from build123d import *

# Parameters (mm, degrees)
BOSS_EXTRUDE1_DEPTH = 25
SKETCH2_R           = 5
SKETCH2_W           = 17.097123546
SKETCH2_H           = 4.020670456
CUT_EXTRUDE1_DEPTH  = 100
BOSS_EXTRUDE2_DEPTH = 50


with BuildPart() as part:
    # Sketch1 → Boss-Extrude1 (new body)
    with BuildSketch(Plane.XY):
        Polygon((-120, 0), (-87.572195572, 56.166604847), (87.572195572, 56.166604847), (120, 0), (126.793465802, 0), (141.793465802, 0), (141.793465802, 5), (122.886751346, 5), (92.427804428, 57.756443607), (90.458946918, 61.166604847), (-90.458946918, 61.166604847), (-122.886751346, 5), (-141.793465802, 5), (-141.793465802, 0), (-126.793465802, 0), align=None)
    extrude(amount=BOSS_EXTRUDE1_DEPTH)

    # Sketch2 → Cut-Extrude1 (cut, symmetric)
    with BuildSketch(Plane(origin=(0, 5, 0), x_dir=(1, 0, 0), z_dir=(0, 1, 0))):
        with Locations((132.340108574, -12.5)):
            Circle(SKETCH2_R)
        with Locations((-132.340108574, -12.5)):
            Circle(SKETCH2_R)
        with Locations((0, -7.118249896)):
            Rectangle(SKETCH2_W, SKETCH2_H)
    extrude(amount=CUT_EXTRUDE1_DEPTH, both=True, mode=Mode.SUBTRACT)

    # Sketch3 → Boss-Extrude2 (add, symmetric)
    with BuildSketch(Plane(origin=(0, 0, 0), x_dir=(0, 0, -1), z_dir=(1, 0, 0))):
        Polygon((-30.808478502, 77.125268372), (-20.547874202, 48.934489749), (-25.246337306, 47.224389032), (-27.125722548, 46.540348745), (-28.493803121, 50.299119228), (-27.5541105, 50.641139372), (-26.52805007, 47.822061509), (-25.588357449, 48.164081653), (-35.164921463, 74.475475035), (-36.104614083, 74.133454891), (-35.078553653, 71.314377029), (-36.018246274, 70.972356886), (-37.386326847, 74.731127369), (-35.506941606, 75.415167656), align=None)
    extrude(amount=BOSS_EXTRUDE2_DEPTH, both=True)


solid = part.part
Verification items for the finished model (mm, model axes). A direction names the side the tool comes from. Coordinates: 2 decimals unless noted, no trailing zeros. Order: outer loops, then holes, each group sorted by start corner. A loop starts at its lowest first (then second) coordinate and runs counter-clockwise, first axis right, second up. Notation, with made-up numbers: M 30.25,-38 L 54.25,-38 A28 ccw 54.25,-8 Z; hole C 46.5,50 d9. An arc over 180 degrees is marked long. One line per item, written item: value. Start each with the question number.
Item 1: Sectioned sample at C-C (y = 22). Enter the section's corners in (x, z), then the cut area to 3 significant figures.
Item 2: Mould release check, pull along X, two halves, no side actions. Record for faces 1 (the flat face through (-104.013, 27.69, 12.325)), 2 (the flat face through (126, 0, 12)), 3 (the flat face through (-141.793, 3, 12)): released by +X, released by -X, zero draft, split by the parting line, or undercut.
Item 3: Sectioned sample at B-B (x = -30). Enter the section's corners in (y, z), then the cut area to 3 significant figures.
Item 4: Scan lines: probe 1 along Y at (x, z) = (52, 14); probe 2 along X at (y, z) = (4, 14.5); probe 3 along Y at (x, z) = (-16, 23.5). Record each from-to range of solid material in increasing order.
Item 5: Gauge pin test, flat ends, axial feed: pin 1 (5 mm diameter, centred on y = 64, z = 33, fed in from -X); pin 2 (2 mm diameter, centred on y = 59, z = 6.5, fed in from +X); pin 3 (5.5 mm diameter, centred on x = -129.5, z = 11.5, fed in from +Y); pin 4 (6 mm diameter, centred on x = -132.34, z = 12.5, fed in from -Y). Record the tip position at first contact, or that the pin passes through.
Item 6: Sectioned sample at D-D (y = 67). Enter the section's corners in (x, z).
Item 7: Access from +Z, -Z, +X, -X, +Y, -Y to the whole of each face (thin tool, end or side, straight path). Record for faces 4 (the flat face through (1, 61.167, 12)), 5 (the flat face through (137, 5, 10)), 6 (the flat face through (0.7, 52.6, 21.88)).
Item 8: Sectioned sample at A-A (z = 12.5). Enter the section's corners in (x, y).
Conclusion:
1. outline: M -113.07,0 L -107.3,0 L -107.3,25 L -113.07,25 Z; M 107.3,0 L 113.07,0 L 113.07,25 L 107.3,25 Z
1. area: 289 mm^2
2. face 1: undercut
2. face 2: zero draft
2. face 3: released by -X
3. outline: M 46.54,27.13 L 48.93,20.55 L 56.17,23.18 L 56.17,0 L 61.17,0 L 61.17,25 L 77.13,30.81 L 74.73,37.39 L 70.97,36.02 L 71.31,35.08 L 74.13,36.1 L 74.48,35.16 L 48.16,25.59 L 47.82,26.53 L 50.64,27.55 L 50.3,28.49 Z
3. area: 280 mm^2
4. probe 1: y = 56.17 to 61.17
4. probe 2: x = -141.79 to -136.92, -127.76 to -117.69, 117.69 to 127.76, 136.92 to 141.79
4. probe 3: y = 47.86 to 61.17
5. pin 1: stops at x = -50
5. pin 2: stops at x = 92.29
5. pin 3: stops at y = 5
5. pin 4: passes through
6. outline: M -50,27.12 L 50,27.12 L 50,32.44 L -50,32.44 Z
7. face 4: -Z, +X, -X, +Y
7. face 5: +Z, -Z, +X, +Y
7. face 6: -Z
8. outline: M -141.79,0 L -137.34,0 L -137.34,5 L -141.79,5 Z; M -127.34,0 L -120,0 L -87.57,56.17 L 87.57,56.17 L 120,0 L 127.34,0 L 127.34,5 L 122.89,5 L 90.46,61.17 L -90.46,61.17 L -122.89,5 L -127.34,5 Z; M 137.34,0 L 141.79,0 L 141.79,5 L 137.34,5 Z
